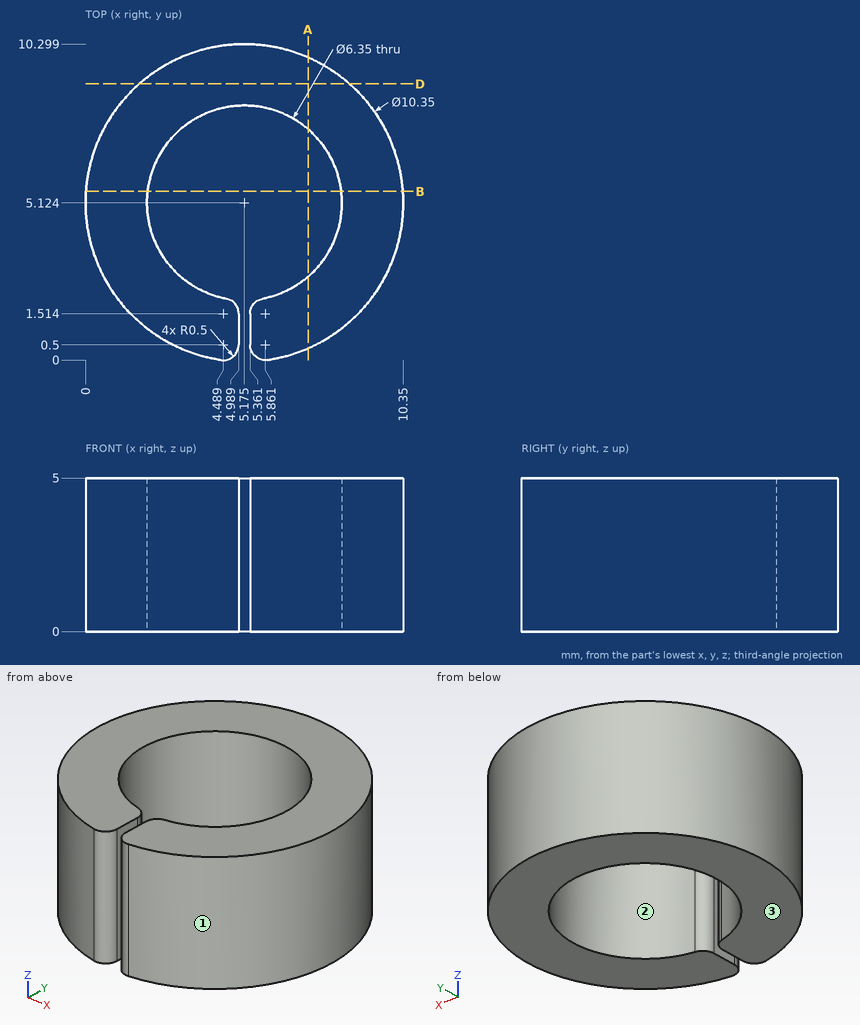
For this review, use the dimensioned drawing (mm, ordinates from the lowest corner) and the shaded views. Round coordinates to 2 decimals unless told otherwise and drop trailing zeros. Write each loop counter-clockwise with the first axis right and the second up, starting at its lowest first coordinate (ties: lowest second). Pieces come first, ordered by that corner, then holes. Notation, with made-up numbers: (38, -36) -> (46, -36) arc R34 ccw to (46, -3) -> close; hole circle Ø2 at (76.5, -18.75). An arc over 180 degrees is marked (long way). Use CSV: the item, a comma, the result in double quotes.
Q1. Consider section B-B (y = 5.5). Give the boundary of the cut face in (x, z), then the cut area to 3 significant figures.
Checks:
outline,"(0.01, 0) -> (2.02, 0) -> (2.02, 5) -> (0.01, 5) -> close; (8.33, 0) -> (10.34, 0) -> (10.34, 5) -> (8.33, 5) -> close"
area,"20.1 mm²"
Q2. Mouldability with a two-part tool opening along X and no side actions: class the marked faces 1, 2 and 3 as released by +X, released by -X, zero draft, split by the parting line, or undercut.
Checks:
face 1,"split by the parting line"
face 2,"undercut"
face 3,"zero draft"
Q3. For pin 1 Ø0.5 at (y, z) = (1, 3.5) entering from +X (1 decimal); pin 2 Ø5.5 at (x, y) = (5.18, 5.12) entering from +Z; pin 3 Ø1.1 at (y, z) = (1, 2.5) entering from -X, all flat-tipped, find the tip position at first contact; note any pin that passes through.
Checks:
pin 1,"x = 8.6"
pin 2,"through"
pin 3,"x = 1.43"
Q4. To check wall thickness, follow probe 1 along X at (y, z) = (5.25, 4.1); probe 2 along X at (y, z) = (6.5, 2.55) (1 decimal); probe 3 along Y at (x, z) = (4, 0.75) (1 decimal). State the ranges of each line that lie inside material, in increasing order. Write a range as [from, to].
Checks:
probe 1,"[0, 2], [8.35, 10.35]"
probe 2,"[0.2, 2.3], [8, 10.2]"
probe 3,"[0.1, 2.2], [8.1, 10.2]"
Q5. Consider section D-D (y = 9). Give the boundary of the cut face in (x, z) (1 decimal), then the cut area to 3 significant figures.
Checks:
outline,"(1.7, 0) -> (8.6, 0) -> (8.6, 5) -> (1.7, 5) -> close"
area,"34.3 mm²"
Q6. Consider section A-A (x = 7.25). Give the boundary of the cut face in (y, z) (1 decimal).
Checks:
outline,"(0.4, 0) -> (2.7, 0) -> (2.7, 5) -> (0.4, 5) -> close; (7.5, 0) -> (9.9, 0) -> (9.9, 5) -> (7.5, 5) -> close"
